from build123d import *

# Parameters (mm, degrees)
HOLE_WIZARD_M6_1_D     = 5
HOLE_WIZARD_M6_1_DEPTH = 17
HOLE_WIZARD_M6_1_TIP   = 1.502151548
CUT_EXTRUDE_1_DEPTH    = 10
CUT_EXTRUDE_2_DEPTH    = 10
CHAMFER_1_SIZE         = 1


with BuildPart() as part:
    # 草图1 → 旋转1 (revolve)
    with BuildSketch(Plane.XY, mode=Mode.PRIVATE) as revolve_1_sk:
        Polygon((0, 0), (0, 17.5), (75, 17.5), (75, 25), (105, 25), (105, 22.5), (140, 22.5), (140, 22.25), (165, 22.25), (165, 22.5), (210, 22.5), (210, 22.25), (235, 22.25), (235, 17.5), (253, 17.5), (253, 0), align=None)
    revolve(revolve_1_sk.sketch.rotate(Axis((0, 0, 0), (1, 0, 0)), 90), axis=Axis((0, 0, 0), (1, 0, 0)))

    # M6 螺纹孔1
    with Locations(Plane(origin=(0, 0, 0), x_dir=(0, 0, -1), z_dir=(-1, 0, 0))):
        with Locations((0, 0)):
            Hole(HOLE_WIZARD_M6_1_D / 2, depth=HOLE_WIZARD_M6_1_DEPTH)
            with Locations((0, 0, -(HOLE_WIZARD_M6_1_DEPTH + HOLE_WIZARD_M6_1_TIP / 2))):  # 118° drill point
                Cone(0, HOLE_WIZARD_M6_1_D / 2, HOLE_WIZARD_M6_1_TIP, mode=Mode.SUBTRACT)

    # 草图4 → 切除-拉伸1 (cut)
    with BuildSketch(Plane.XY.offset(17)):
        with BuildLine():
            Line((113, 7), (132, 7))
            ThreePointArc((132, 7), (139, 0), (132, -7))
            Line((132, -7), (113, -7))
            ThreePointArc((113, -7), (106, 0), (113, 7))
        make_face()
        with BuildLine():
            Line((173, 7), (202, 7))
            ThreePointArc((202, 7), (209, 0), (202, -7))
            Line((202, -7), (173, -7))
            ThreePointArc((173, -7), (166, 0), (173, 7))
        make_face()
    extrude(amount=CUT_EXTRUDE_1_DEPTH, mode=Mode.SUBTRACT)

    # 草图5 → 切除-拉伸2 (cut)
    with BuildSketch(Plane.XY.offset(12.5)):
        with BuildLine():
            Line((8, 5), (38, 5))
            ThreePointArc((38, 5), (43, 0), (38, -5))
            Line((38, -5), (8, -5))
            ThreePointArc((8, -5), (3, 0), (8, 5))
        make_face()
    extrude(amount=CUT_EXTRUDE_2_DEPTH, mode=Mode.SUBTRACT)

    # 倒角1
    chamfer_1_edges = [part.edges().sort_by_distance(p)[0] for p in [
        (253, 0, -17.5),
        (0, 0, -17.5),
    ]]
    chamfer(chamfer_1_edges, length=CHAMFER_1_SIZE)


solid = part.part
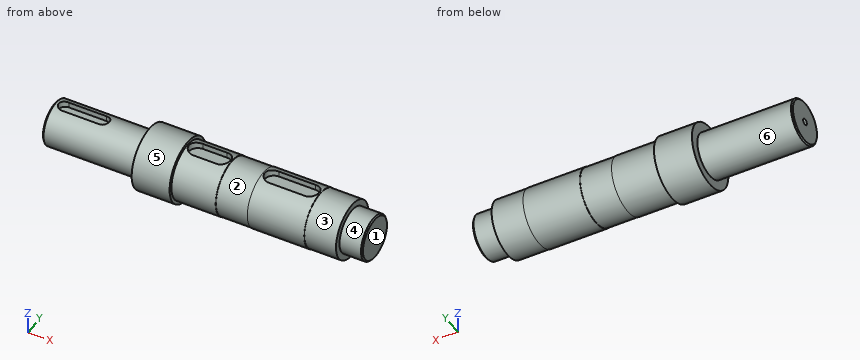
Build history of the part. All positions in model axes, mm. Face numbers are marked on the shaded views. A direction names the side the tool comes from. Give positions to 0.01 mm unless a question says otherwise; leave off trailing zeros. Order: outer loops, then holes, each group sorted by start corner. A loop starts at its lowest first (then second) coordinate and runs counter-clockwise, first axis right, second up. Notation, with made-up numbers: M 40.5,-33.75 L 72.5,-33.75 A32 cw 72.5,1.25 Z; hole C 73,25 d8. An arc over 180 degrees is marked long. Put each result on its own line as item: value.
Item 1: Wall check: probe 1 along Y at (x, z) = (9.75, 0); probe 2 along X at (y, z) = (9, 18); probe 3 along X at (y, z) = (21, -13.5). Give the ranges that are in metal, low to high.
Results are:
probe 1: -17.5 to -2.5, 2.5 to 17.5
probe 2: 75 to 235
probe 3: 75 to 105
Item 2: Drop flat-ended pins along their axis: pin 1 Ø7 at (x, y) = (197.5, -2) entering from +Z; pin 2 Ø5 at (x, z) = (140, 2.5) entering from -Y; pin 3 Ø4 at (x, z) = (202.5, 5) entering from +Y. Give the stop position or say it passes through.
Results are:
pin 1: z = 17
pin 2: y = -22.5
pin 3: y = 22.3
Item 3: Pull direction X, two halves, no side cores. Call the marked faces 1, 2 and 3: +X half, -X half, draft (parallel to the pull), parting line (faces both ways), or undercut.
Results are:
face 1: +X half
face 2: undercut
face 3: draft
Item 4: Cut at A-A on x = 228. Write the cut outline in (y, z).
Results are:
outline: C 0,0 d44.5
Item 5: Which spindle directions (+Z, -Z, +X, -X, +Y, -Y) get a long thin tool onto all of the face, cutting with end or side? Do the marked faces 4, 5 and 6. Say none if no direction does.
Results are:
face 4: +X
face 5: +X, -X
face 6: -X
Item 6: Cut at B-B on x = 87. Write the cut outline in (y, z).
Results are:
outline: C 0,0 d50
